Autodesk Inventor part; units mm, degrees
ref_plane "YZ Plane" through (0, 0, 0) normal (1, 0, 0) x (0, 1, 0)
ref_plane "XZ Plane" through (0, 0, 0) normal (0, 1, 0) x (-1, 0, 0)
ref_plane "XY Plane" through (0, 0, 0) normal (0, 0, 1) x (1, 0, 0)
sketch "スケッチ1" plane through (0, 0, 0) normal (0, 1, 0) x (-1, 0, 0)
  circle A0 centre (0, 0) radius 38
  dimension "d0" = 76
extrude "押し出し1" add sketch "スケッチ1" along normal blind 36.5
sketch "スケッチ3" plane through (0, 36.5, 0) normal (0, 1, 0) x (1, 0, 0)
  circle A0 centre (0, 0) radius 20.25
  dimension "d6" = 40.5
extrude "押し出し3" cut sketch "スケッチ3" against normal blind 6.5
sketch "スケッチ4" plane through (0, 36.5, 0) normal (0, 1, 0) x (1, 0, 0)
  circle A0 centre (0, 0) radius 20.25
extrude "押し出し4" add sketch "スケッチ4" against normal blind 2
sketch "スケッチ6" plane through (0, 0, 0) normal (0, -1, 0) x (1, 0, 0)
  circle A0 centre (0, 0) radius 12.25
  dimension "d13" = 24.5
extrude "押し出し5" cut sketch "スケッチ6" against normal through all
sketch "スケッチ7" plane through (0, 0, 0) normal (1, 0, 0) x (0, 1, 0)
  line L0 (34.5, -20.25) -> (34.5, 20.25)
  line L1 (30, 20.25) -> (30, -20.25)
  line L2 (34.5, 20.25) -> (30, 20.25)
  line L3 (30, 20.25) -> (30, -20.25)
  line L4 (30, -20.25) -> (34.5, -20.25)
  line L5 (34.5, -20.25) -> (34.5, 20.25)
  point P0 (0, 0)
extrude "押し出し6" cut sketch "スケッチ7" along normal through all
sketch "スケッチ8" plane through (0, 0, 0) normal (1, 0, 0) x (0, 1, 0)
  line L0 (36.5, 12.25) -> (36.5, -12.25)
  line L1 (34.5, -12.25) -> (34.5, 12.25)
  line L2 (36.5, 12.25) -> (34.5, 12.25)
  line L3 (34.5, 12.25) -> (34.5, -12.25)
  line L4 (34.5, -12.25) -> (36.5, -12.25)
  line L5 (36.5, -12.25) -> (36.5, 12.25)
  point P0 (0, 0)
extrude "押し出し7" cut sketch "スケッチ8" along normal through all
sketch "スケッチ10" plane through (0, 0, 0) normal (0, -1, 0) x (1, 0, 0)
  circle A0 centre (0, 0) radius 12.25
extrude "押し出し9" add sketch "スケッチ10" against normal blind 30
sketch "スケッチ11" plane through (0, 0, 0) normal (0, -1, 0) x (1, 0, 0)
  circle A0 centre (0, 0) radius 11
  dimension "d25" = 22
extrude "押し出し10" cut sketch "スケッチ11" against normal through all
sketch "スケッチ13" plane through (0, 0, 0) normal (0, 0, 1) x (1, 0, 0)
  line L0 (-11, 30) -> (11, 30)
  line L1 (0, 30) -> (0, 28) construction
  line L2 (0, 28) -> (-12.75, 28)
  line L3 (-12.75, 28) -> (-12.75, 24)
  line L4 (-12.75, 24) -> (0, 24)
  line L5 (0, 24) -> (0, 28)
  line L6 (0, -7.3) -> (0, 43.8)
  point P0 (0, 0)
  dimension "d29" = 2
  dimension "d30" = 12.75
  dimension "d31" = 4
revolve "回転2" cut sketch "スケッチ13" angle 360 about axis through (0, -10, 0) along (0, -1, 0)
sketch "スケッチ14" plane through (0, 0, 0) normal (1, 0, 0) x (0, 1, 0)
  line L0 (28, 12.75) -> (24, 12.75)
  line L1 (28, -12.75) -> (24, -12.75)
  line L2 (24, 12.75) -> (28, 12.75)
  line L3 (28, 12.75) -> (28, -12.75)
  line L4 (28, -12.75) -> (24, -12.75)
  line L5 (24, -12.75) -> (24, 12.75)
  point P0 (0, 0)
extrude "押し出し11" cut sketch "スケッチ14" against normal through all
sketch "スケッチ15" plane through (0, 0, 0) normal (1, 0, 0) x (0, 1, 0)
  line L0 (24, 0) -> (24, -5.5)
  line L1 (24, -5.5) -> (28, -5.5)
  line L2 (28, -5.5) -> (28, 0)
  line L3 (24, 0) -> (24, 5.5)
  line L4 (24, 5.5) -> (28, 5.5)
  line L5 (28, 5.5) -> (28, 0)
  point P0 (0, 0)
  dimension "d35" = 4
  dimension "d36" = 5.5
extrude "押し出し12" cut sketch "スケッチ15" along normal through all
sketch "スケッチ16" plane through (0, 0, 0) normal (0, -1, 0) x (1, 0, 0)
  circle A0 centre (0, 0) radius 38
extrude "押し出し13" add sketch "スケッチ16" along normal blind 8
sketch "スケッチ17" plane through (0, -8, 0) normal (0, -1, 0) x (1, 0, 0)
  circle A0 centre (0, 0) radius 11
extrude "押し出し14" cut sketch "スケッチ17" against normal through all
sketch "スケッチ19" plane through (0, -8, 0) normal (0, -1, 0) x (1, 0, 0)
  circle A0 centre (0, 0) radius 36.25
  dimension "d44" = 72.5
extrude "押し出し15" cut sketch "スケッチ19" against normal blind 30
properties part number "lens-holder_LIBS" material "ABS プラスチック"
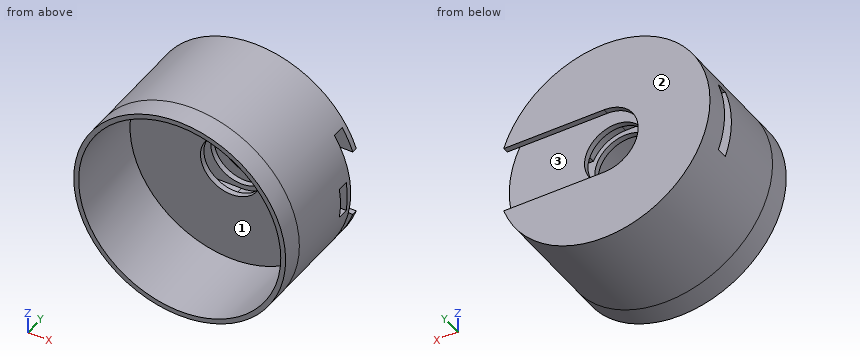
Verification items for the finished model (mm, model axes). Face numbers are marked on the shaded views. Coordinates: 2 decimals unless noted, no trailing zeros. Loops run counter-clockwise (first coordinate to the right, second up) from the corner with the lowest first, then second, coordinate; pieces in that order, holes last. Notation, with made-up numbers: (58, 79.25) -> (94, 79.25) arc R32 cw to (94, 109.25) -> close; hole circle Ø11 at (-17, 19). An arc over 180 degrees is marked (long way). Answer in a Markdown table with one row per item.
1) Section check C-C (z = -9.5). Record the cut outline in (x, y), and give its area (3 significant figures).
The answers:
| item | result |
|---|---|
| outline | (-36.79, -8) -> (-34.98, -8) -> (-34.98, 22) -> (-5.55, 22) -> (-5.55, 24) -> (-36.79, 24) -> close; (-36.79, 28) -> (-5.55, 28) -> (-5.55, 30) -> (-17.88, 30) -> (-17.88, 34.5) -> (-7.73, 34.5) -> (-7.73, 36.5) -> (-36.79, 36.5) -> close; (5.55, 22) -> (34.98, 22) -> (34.98, -8) -> (36.79, -8) -> (36.79, 30) -> (5.55, 30) -> (5.55, 28) -> (8.5, 28) -> (8.5, 24) -> (5.55, 24) -> close |
| area | 615 mm2 |
2) Scan lines: line 1 along Y through (x, z) = (-12, 10.5); line 2 along Z through (x, y) = (0, 29); line 3 along Y through (x, z) = (-11, 1.5). Record each from-to range of solid material in increasing order. Write a range as from..to.
The answers:
| item | result |
|---|---|
| line 1 | y = 22..24, 28..30, 34.5..36.5 |
| line 2 | z = -38..-11, 11..38 |
| line 3 | y = 22..24, 28..30 |
3) Depth check by flat-ended pin: P1, Ø2, axis at x = 21.5, y = 25, coming from the +Z side; P2, Ø4, axis at x = 28, y = 9, coming from the +Z side; P3, Ø3, axis at x = 5, z = -18, coming from the -Y side. Enter the tip coordinate at first touch or a pass-through.
The answers:
| item | result |
|---|---|
| P1 | stops at z = 32 |
| P2 | stops at z = 27.71 |
| P3 | stops at y = 22 |
4) Section check A-A (y = 25). Record the cut outline in (x, z), and give its area (3 significant figures).
The answers:
| item | result |
|---|---|
| outline | (-35.8, -12.75) arc R38 ccw to (37.6, -5.5) -> (11.5, -5.5) arc R12.75 cw to (0, -12.75) -> close; (-35.8, 12.75) -> (0, 12.75) arc R12.75 cw to (11.5, 5.5) -> (37.6, 5.5) arc R38 ccw to start |
| area | 3,050 mm2 |
5) Draft check along Y on the marked faces 1, 2 and 3. Enter one of: released by +Y, released by -Y, zero draft, split by the parting line, or undercut.
The answers:
| item | result |
|---|---|
| face 1 | released by -Y |
| face 2 | released by +Y |
| face 3 | undercut |
6) Section check D-D (x = -22.5). Record the cut outline in (y, z), and give its area (3 significant figures).
The answers:
| item | result |
|---|---|
| outline | (-8, -30.62) -> (36.5, -30.62) -> (36.5, 30.62) -> (-8, 30.62) -> (-8, 28.42) -> (22, 28.42) -> (22, -28.42) -> (-8, -28.42) -> close; hole (24, -12.75) -> (28, -12.75) -> (28, 12.75) -> (24, 12.75) -> close |
| area | 918 mm2 |
7) Section check B-B (z = 0). Record the cut outline in (x, y), and give its area (3 significant figures).
The answers:
| item | result |
|---|---|
| outline | (-38, -8) -> (-36.25, -8) -> (-36.25, 22) -> (-11, 22) -> (-11, 24) -> (-38, 24) -> close; (-38, 28) -> (-11, 28) -> (-11, 30) -> (-20.25, 30) -> (-20.25, 34.5) -> (-12.25, 34.5) -> (-12.25, 36.5) -> (-38, 36.5) -> close; (11, 22) -> (36.25, 22) -> (36.25, -8) -> (38, -8) -> (38, 24) -> (11, 24) -> close; (11, 28) -> (38, 28) -> (38, 30) -> (11, 30) -> close |
| area | 452 mm2 |
